Design review of the part built by this model. Coordinates are the model's own, in mm. Round coordinates to 2 decimals unless told otherwise and drop trailing zeros. Order: outer loops, then holes, each group sorted by start corner. A loop starts at its lowest first (then second) coordinate and runs counter-clockwise, first axis right, second up.
from build123d import *

# Parameters (mm, degrees)
ESQUISSE1_R                = 18
ESQUISSE1_R_2              = 15
EXTRU_MINCE1_DEPTH         = 635
ESQUISSE2_R                = 3
ENL_V_MAT_EXTRU_1_DEPTH    = 30
R_P_TITION_LIN_AIRE1_COUNT = 4
R_P_TITION_LIN_AIRE1_PITCH = 140


with BuildPart() as part:
    # Esquisse1 → Extru.-Mince1 (new body)
    with BuildSketch(Plane.XY):
        Circle(ESQUISSE1_R)
        Circle(ESQUISSE1_R_2, mode=Mode.SUBTRACT)
    extrude(amount=EXTRU_MINCE1_DEPTH)

    # Esquisse2 → Enl_v. mat.-Extru.1 (cut, symmetric)
    with BuildSketch(Plane(origin=(0, 0, 0), x_dir=(1, 0, 0), z_dir=(0, 1, 0))):
        with Locations(Location((0, -108, 0), (0, 0, 90))):
            Circle(ESQUISSE2_R)
    enl_v_mat_extru_1 = extrude(amount=ENL_V_MAT_EXTRU_1_DEPTH, both=True, mode=Mode.SUBTRACT)

    # R_p_tition lin_aire1: Enl_v. mat.-Extru.1 ×4
    with Locations(*[(0, 0, i * R_P_TITION_LIN_AIRE1_PITCH) for i in range(1, R_P_TITION_LIN_AIRE1_COUNT)]):
        add(enl_v_mat_extru_1, mode=Mode.SUBTRACT)


solid = part.part
1) To check wall thickness, follow line 1 along X through (y, z) = (1, 540.5); line 2 along Y through (x, z) = (5, 495); line 3 along X through (y, z) = (16.5, 108). State the ranges of each line that lie inside material, in increasing order.
Results:
line 1: x = -17.97 to -14.97, 14.97 to 17.97
line 2: y = -17.29 to -14.14, 14.14 to 17.29
line 3: x = -7.19 to -3, 3 to 7.19
2) Take a section at C-C on z = 257. Give the boundary of the cut face in (x, y).
Results:
outline: circle Ø36 at (0, 0); hole circle Ø30 at (0, 0)
3) Take a section at A-A on y = -8. Give the boundary of the cut face in (x, z).
Results:
outline: (-16.12, 0) - (-12.69, 0) - (-12.69, 635) - (-16.12, 635) - close; (12.69, 0) - (16.12, 0) - (16.12, 635) - (12.69, 635) - close
4) Clearance check with flat-ended pins moving along their axes: P1, Ø4, axis at y = -3, z = 257, coming from the +X side; P2, Ø1, axis at x = -6.5, y = 13.5, coming from the -Z side; P3, Ø1.5, axis at y = -6, z = 275.5, coming from the -X side; P4, Ø1.5, axis at x = -2.5, z = 284.5, coming from the +Y side. State where each tip first meets the part, or that it passes through.
Results:
P1: stops at x = 17.97
P2: stops at z = 0
P3: stops at x = -17.22
P4: stops at y = 17.91
5) Take a section at B-B on x = 9. Give the boundary of the cut face in (y, z).
Results:
outline: (-15.59, 0) - (-12, 0) - (-12, 635) - (-15.59, 635) - close; (12, 0) - (15.59, 0) - (15.59, 635) - (12, 635) - close
